```python
from build123d import *

# Parameters (mm, degrees)
F0_W      = 80
F0_H      = 122.4
F1_DEPTH  = 6
F2_W      = 76.1
F2_H      = 26.1
F2_W_2    = 74.6
F2_H_2    = 24.6
F3_DEPTH  = 1.2
F4_DEPTH  = 6.001
F6_D      = 3
F6_DEPTH  = 15
F6_TIP    = 0.9012909285
F8_D      = 3
F8_DEPTH  = 15
F8_TIP    = 0.9012909285
F9_R      = 2
F11_DEPTH = 6.001
F12_W     = 0.5
F12_H     = 0.5
F13_DEPTH = 4.8010001
F15_DEPTH = 6.0010001
F16_W     = 0.5
F16_H     = 0.5
F17_DEPTH = 4.8010001


# Not quite as in the source:
# - the program builds the solid bodies; features that only make, move or delete a surface that nothing else refers to are left out


with BuildPart() as f1:
    # F0 (on Top) → F1 (new body)
    with BuildSketch(Plane.XY):
        Rectangle(F0_W, F0_H)
    extrude(amount=F1_DEPTH)

    # F2 (on face) → F3 (cut)
    with BuildSketch(Plane.XY.offset(6)):
        with Locations((0, -45.15)):
            Rectangle(F2_W, F2_H)
        with Locations((0, -45.15)):
            Rectangle(F2_W_2, F2_H_2, mode=Mode.SUBTRACT)
        with Locations((0, -16.05)):
            Rectangle(F2_W, F2_H)
        with Locations((0, -16.05)):
            Rectangle(F2_W_2, F2_H_2, mode=Mode.SUBTRACT)
        with Locations((0, 16.05)):
            Rectangle(F2_W, F2_H)
        with Locations((0, 16.05)):
            Rectangle(F2_W_2, F2_H_2, mode=Mode.SUBTRACT)
        with Locations((0, 45.15)):
            Rectangle(F2_W, F2_H)
        with Locations((0, 45.15)):
            Rectangle(F2_W_2, F2_H_2, mode=Mode.SUBTRACT)
    extrude(amount=-F3_DEPTH, mode=Mode.SUBTRACT)

    # F4 (cut, through all): faces of the model
    f4_faces = [f1.faces().sort_by_distance(p)[0] for p in [
        (0, -45.15, 6),
        (0, -16.05, 6),
        (0, 16.05, 6),
        (0, 45.15, 6),
    ]]
    extrude(f4_faces, amount=-F4_DEPTH, mode=Mode.SUBTRACT)

    # F6
    with Locations(Plane.YZ.offset(40)):
        with Locations((-30.6025246664, 2.9744678242), (30.6, 2.9233971525)):
            Hole(F6_D / 2, depth=F6_DEPTH)
            with Locations((0, 0, -(F6_DEPTH + F6_TIP / 2))):  # 118° drill point
                Cone(0, F6_D / 2, F6_TIP, mode=Mode.SUBTRACT)

    # F8
    with Locations(Plane(origin=(-40, 0, 0), x_dir=(0, -1, 0), z_dir=(-1, 0, 0))):
        with Locations((30.6188296527, 2.9554700013), (-30.6144393981, 2.9124866705)):
            Hole(F8_D / 2, depth=F8_DEPTH)
            with Locations((0, 0, -(F8_DEPTH + F8_TIP / 2))):  # 118° drill point
                Cone(0, F8_D / 2, F8_TIP, mode=Mode.SUBTRACT)

    # F9
    f9_edges = [f1.edges().sort_by_distance(p)[0] for p in [
        (-40, -61.2, 3),
        (40, -61.2, 3),
        (40, 61.2, 3),
        (-40, 61.2, 3),
    ]]
    fillet(f9_edges, radius=F9_R)

    # F10 (on face) → F11 (cut, through all)
    with BuildSketch(Plane.XY.offset(6)):
        with BuildLine():
            Line((-38.3, -32.6), (-38.05, -32.6))
            Line((-38.05, -32.6), (-38.05, -32.1))
            Line((-38.05, -32.1), (-37.55, -32.1))
            Line((-37.55, -32.1), (-37.55, -31.85))
            ThreePointArc((-37.55, -31.85), (-37.6232233047, -31.6732233047), (-37.8, -31.6))
            Line((-37.8, -31.6), (-38.3, -31.6))
            ThreePointArc((-38.3, -31.6), (-38.4767766953, -31.6732233047), (-38.55, -31.85))
            Line((-38.55, -31.85), (-38.55, -32.35))
            ThreePointArc((-38.55, -32.35), (-38.4767766953, -32.5267766953), (-38.3, -32.6))
        make_face()
    extrude(amount=-F11_DEPTH, mode=Mode.SUBTRACT)

    # F12 (on face) → F13 (cut, through all)
    with BuildSketch(Plane.XY.offset(4.8)):
        with Locations((-37.8, -32.35)):
            Rectangle(F12_W, F12_H)
    extrude(amount=-F13_DEPTH, mode=Mode.SUBTRACT)

    # F14 (on face) → F15 (cut, through all)
    with BuildSketch(Plane.XY.offset(6)):
        with BuildLine():
            Line((37.8, -58.7), (38.3, -58.7))
            ThreePointArc((38.3, -58.7), (38.4767766953, -58.6267766953), (38.55, -58.45))
            Line((38.55, -58.45), (38.55, -57.95))
            ThreePointArc((38.55, -57.95), (38.4767766953, -57.7732233047), (38.3, -57.7))
            Line((38.3, -57.7), (38.05, -57.7))
            Line((38.05, -57.7), (38.05, -58.2))
            Line((38.05, -58.2), (37.55, -58.2))
            Line((37.55, -58.2), (37.55, -58.45))
            ThreePointArc((37.55, -58.45), (37.6232233047, -58.6267766953), (37.8, -58.7))
        make_face()
    extrude(amount=-F15_DEPTH, mode=Mode.SUBTRACT)

    # F16 (on face) → F17 (cut, through all)
    with BuildSketch(Plane.XY.offset(4.8)):
        with Locations((37.8, -57.95)):
            Rectangle(F16_W, F16_H)
    extrude(amount=-F17_DEPTH, mode=Mode.SUBTRACT)


solid = f1.part
```
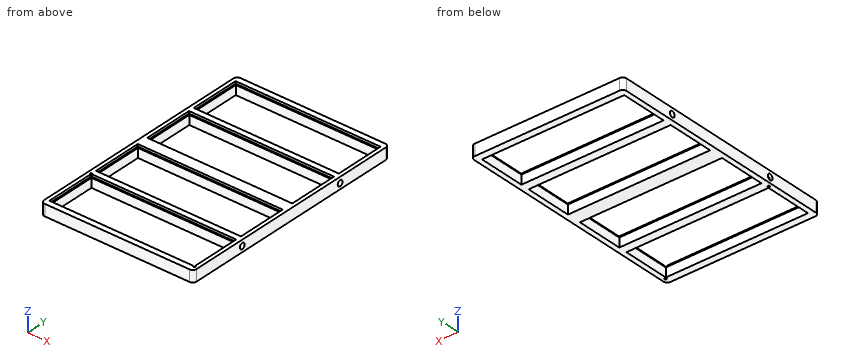
Model file for the job. Use its own axes, mm. Coordinates: 2 decimals unless noted, no trailing zeros. Order: outer loops, then holes, each group sorted by start corner. A loop starts at its lowest first (then second) coordinate and runs counter-clockwise, first axis right, second up. Notation, with made-up numbers: (77, 39) -> (83, 39) arc R24 ccw to (83, 50) -> close; hole circle Ø10 at (70, 85.25). An arc over 180 degrees is marked (long way). Answer as a JSON object with one key per item and string values. Group by question number.
1) Cut at B-B, the plane x = 30.5. Count the separate pieces of the cut face and the enclosed holes in it, then the cut area to 3 significant figures.
2) Drill centre lines: L1, parallel to Y at x = -16, z = 2.25; L2, parallel to X at y = 38.5, z = 5; L3, parallel to X at y = -23.5, z = 3. Where is each one in solid material? Low to high.
3) Cut at A-A, the plane y = -16.5. Write the cut outline in (x, z).
Check values:
{
 "1": {"separate pieces": "5", "enclosed holes": "2", "area": "123 mm²"},
 "2": {"L1": "y = -61.2 to -57.45, -32.85 to -28.35, -3.75 to 3.75, 28.35 to 32.85, 57.45 to 61.2", "L2": "x = -40 to -38.05, 38.05 to 40", "L3": "x = -40 to -37.3, 37.3 to 40"},
 "3": {"outline": "(-40, 0) -> (-37.3, 0) -> (-37.3, 4.8) -> (-38.05, 4.8) -> (-38.05, 6) -> (-40, 6) -> close; (37.3, 0) -> (40, 0) -> (40, 6) -> (38.05, 6) -> (38.05, 4.8) -> (37.3, 4.8) -> close"}
}
